Work out the finished part from the listing and answer in its coordinate system (mm). Face numbers are marked on the shaded views. A direction names the side the tool comes from. Coordinates: 2 decimals unless noted, no trailing zeros. Loops run counter-clockwise (first coordinate to the right, second up) from the corner with the lowest first, then second, coordinate; pieces in that order, holes last. Notation, with made-up numbers: (60.25, 46) - (82.25, 46) arc R3 ccw to (82.25, 50) - close; hole circle Ø2 at (88, 20). An arc over 180 degrees is marked (long way). Write each question's results on one line, items separated by ' | '. Start each with the question number.
1. A cutting plane is placed at C-C on y = 5. Determine the outline of the cut face in (x, z).
2. A cutting plane is placed at B-B on x = 53. Determine the outline of the cut face in (y, z).
3. Which of the six approach directions +Z, -Z, +X, -X, +Y, -Y give full straight-line access (tool end or side, diameter ignored) to the marked faces 5, 6 and 7?
4. Find the intervals of material crossed by line 1 along Y through (x, z) = (62.6, 1.15); line 2 along X through (y, z) = (7, 3.5); line 3 along Y through (x, z) = (47.5, 0.7), in increasing order. Write a range as [from, to].
5. Each of these flat-tipped pins is pushed along its axis until it touches: P1, Ø2, axis at x = 14, z = 2.5, coming from the +Y side; P2, Ø2, axis at y = 20, z = 2.5, coming from the -X side; P3, Ø4, axis at x = 62.6, y = 12, coming from the +Z side; P4, Ø2, axis at y = 20.5, z = 2, coming from the +X side. Where does it stop, or does it pass through?
6. A cutting plane is placed at A-A on y = 23.5. Determine the outline of the cut face in (x, z).
7. A cutting plane is placed at D-D on x = 62.6. Determine the outline of the cut face in (y, z), then the cut area to 3 significant figures.
8. Determine the mould class of the marked faces 1, 2, 3 and 4 for opening direction X: released by +X, released by -X, zero draft, split by the parting line, or undercut.
from build123d import *

# Parameters (mm, degrees)
SKETCH_1_R      = 1.6
EXTRUDE_1_DEPTH = 4
FILLET_1_R      = 2


with BuildPart() as part:
    # 草图1 → 凸台-拉伸1 (new body)
    with BuildSketch(Plane.XY):
        Polygon((0, 0), (66.6, 0), (66.6, 16), (42.3, 16), (42.3, 31), (24.3, 31), (24.3, 16), (0, 16), align=None)
        with Locations((4, 4)):
            Circle(SKETCH_1_R, mode=Mode.SUBTRACT)
        with Locations((4, 12)):
            Circle(SKETCH_1_R, mode=Mode.SUBTRACT)
        with Locations(Location((62.6, 12, 0), (0, 0, 180))):
            Circle(SKETCH_1_R, mode=Mode.SUBTRACT)
        with Locations(Location((62.6, 4, 0), (0, 0, 180))):
            Circle(SKETCH_1_R, mode=Mode.SUBTRACT)
        Polygon((8, 12), (28.3, 12), (28.3, 27), (38.3, 27), (38.3, 12), (58.6, 12), (58.6, 4), (8, 4), align=None, mode=Mode.SUBTRACT)
    extrude(amount=EXTRUDE_1_DEPTH)

    # 圆角1
    fillet_1_edges = [part.edges().sort_by_distance(p)[0] for p in [
        (0, 16, 2),
        (24.3, 16, 2),
        (24.3, 31, 2),
        (42.3, 31, 2),
        (42.3, 16, 2),
        (66.6, 16, 2),
        (66.6, 0, 2),
        (0, 0, 2),
        (58.6, 4, 2),
        (58.6, 12, 2),
        (38.3, 12, 2),
        (38.3, 27, 2),
        (28.3, 27, 2),
        (28.3, 12, 2),
        (8, 12, 2),
        (8, 4, 2),
    ]]
    fillet(fillet_1_edges, radius=FILLET_1_R)


solid = part.part
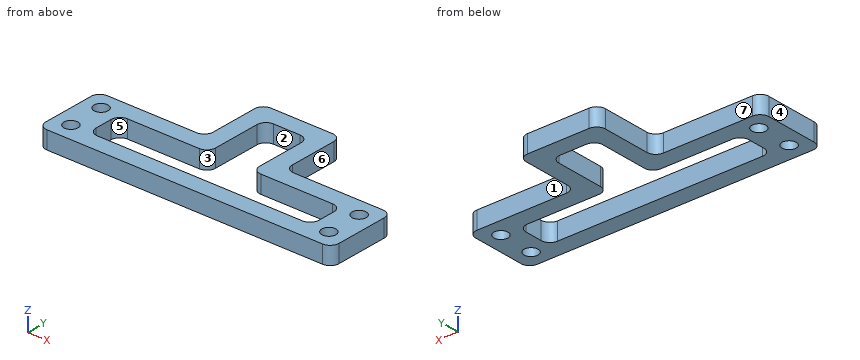
Values:
1) outline: (0, 0) - (2.75, 0) - (2.75, 4) - (0, 4) - close; (5.25, 0) - (8.27, 0) - (8.27, 4) - (5.25, 4) - close; (58.33, 0) - (61.35, 0) - (61.35, 4) - (58.33, 4) - close; (63.85, 0) - (66.6, 0) - (66.6, 4) - (63.85, 4) - close
2) outline: (0, 0) - (4, 0) - (4, 4) - (0, 4) - close; (12, 0) - (16, 0) - (16, 4) - (12, 4) - close
3) face 5: +Z, -Z | face 6: +Z, -Z, +X, +Y | face 7: +Z, -Z, -X, +Y
4) line 1: [0, 2.4], [5.6, 10.4], [13.6, 16] | line 2: [0, 8], [58.6, 66.6] | line 3: [0, 4], [12, 16]
5) P1: y = 16 | P2: x = 24.3 | P3: z = 4 | P4: x = 42.3
6) outline: (24.3, 0) - (28.3, 0) - (28.3, 4) - (24.3, 4) - close; (38.3, 0) - (42.3, 0) - (42.3, 4) - (38.3, 4) - close
7) outline: (0, 0) - (2.4, 0) - (2.4, 4) - (0, 4) - close; (5.6, 0) - (10.4, 0) - (10.4, 4) - (5.6, 4) - close; (13.6, 0) - (16, 0) - (16, 4) - (13.6, 4) - close | area: 38.4 mm^2
8) face 1: zero draft | face 2: undercut | face 3: undercut | face 4: released by -X
